Drawing for the job (mm, zero at the part's lowest x, y, z). A direction names the side the tool comes from. Round coordinates to 2 decimals unless told otherwise and drop trailing zeros. Write each loop counter-clockwise with the first axis right and the second up, starting at its lowest first coordinate (ties: lowest second). Pieces come first, ordered by that corner, then holes.
Item 1: 3-axis set-ups, long thin cutter, end or side, ignore diameter. For the marked faces 1, 2, 3 and 4: which of +Z, -Z, +X, -X, +Y, -Y reach the whole face in a straight line?
Item 2: Band-saw the part on D-D, the plane z = 16. Write the cut outline in (x, y), then the cut area to 3 significant figures.
Item 3: Wall check: probe 1 along X at (y, z) = (1.3, 37); probe 2 along Z at (x, y) = (3.8, 0.7); probe 3 along X at (y, z) = (9.5, 37.5). Give the ranges that are in metal, low to high.
Item 4: Mould opens along Z. For the marked faces 5, 6 and 7 say: +Z half, -Z half, draft (parallel to the pull), parting line (faces both ways), or undercut.
Item 5: Band-saw the part on A-A, the plane z = 3. Write the cut outline in (x, y).
Item 6: Drop flat-ended pins along their axis: pin 1 Ø5 at (x, z) = (35, 27.5) entering from -Y; pin 2 Ø6 at (x, z) = (44, 10) entering from +Y; pin 3 Ø2 at (x, y) = (40.5, 3.5) entering from -Z; pin 4 Ø6 at (y, z) = (5.5, 20) entering from -X. Give the stop position or say it passes through.
Item 7: Band-saw the part on B-B, the plane y = 7. Write the cut outline in (x, z), then the cut area to 3 significant figures.
Item 8: Band-saw the part on C-C, the plane x = 3.8. Write the cut outline in (y, z), then the cut area to 3 significant figures.
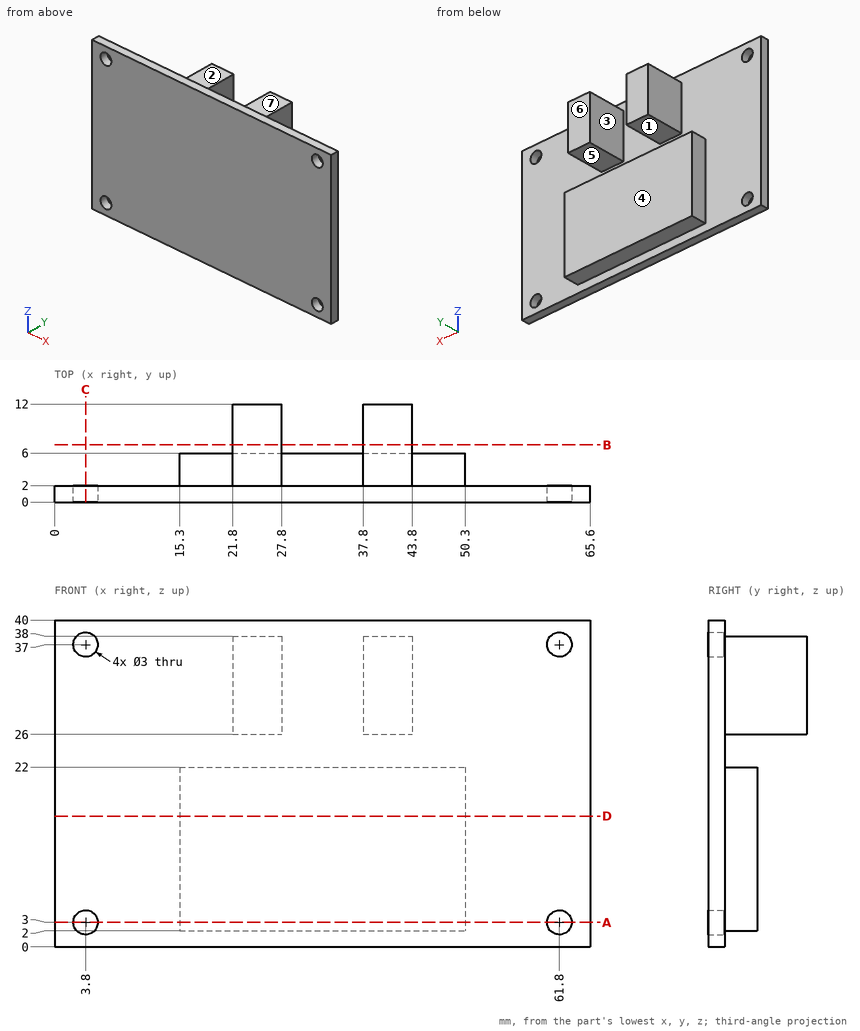
Results:
1. face 1: +X, -X, +Y
1. face 2: +Z, +X, -X, +Y
1. face 3: +Z, +Y
1. face 4: -Z, +X, -X, +Y
2. outline: (0, 0) - (65.6, 0) - (65.6, 2) - (50.3, 2) - (50.3, 6) - (15.3, 6) - (15.3, 2) - (0, 2) - close
2. area: 271 mm2
3. probe 1: x = 0 to 2.3, 5.3 to 60.3, 63.3 to 65.6
3. probe 2: z = 0 to 1.5, 4.5 to 35.5, 38.5 to 40
3. probe 3: x = 21.8 to 27.8, 37.8 to 43.8
4. face 5: undercut
4. face 6: draft
4. face 7: +Z half
5. outline: (0, 0) - (2.3, 0) - (2.3, 2) - (0, 2) - close; (5.3, 0) - (60.3, 0) - (60.3, 2) - (50.3, 2) - (50.3, 6) - (15.3, 6) - (15.3, 2) - (5.3, 2) - close; (63.3, 0) - (65.6, 0) - (65.6, 2) - (63.3, 2) - close
6. pin 1: stops at y = 0
6. pin 2: stops at y = 6
6. pin 3: stops at z = 2
6. pin 4: stops at x = 15.3
7. outline: (21.8, 26) - (27.8, 26) - (27.8, 38) - (21.8, 38) - close; (37.8, 26) - (43.8, 26) - (43.8, 38) - (37.8, 38) - close
7. area: 144 mm2
8. outline: (0, 0) - (2, 0) - (2, 1.5) - (0, 1.5) - close; (0, 4.5) - (2, 4.5) - (2, 35.5) - (0, 35.5) - close; (0, 38.5) - (2, 38.5) - (2, 40) - (0, 40) - close
8. area: 68.0 mm2
